Work out the finished part from the listing and answer in its coordinate system (mm). A direction names the side the tool comes from. Give positions to 0.01 mm unless a question says otherwise; leave off trailing zeros. Write each loop counter-clockwise with the first axis right and the second up, starting at its lowest first coordinate (ties: lowest second). Pieces come first, ordered by that corner, then holes.
1) Find section C-C (y = 5). Determine the outline of the cut face in (x, z).
2) Find section B-B (x = 13.75). Determine the outline of the cut face in (y, z), plus the area to 3 significant figures.
3) Find section D-D (x = 18.25). Determine the outline of the cut face in (y, z).
4) Straight lines are drawn through the part: probe 1 along Y at (x, z) = (15, 15.5); probe 2 along Y at (x, z) = (22.25, 23); probe 3 along Z at (x, y) = (18.8, 7.5). For each, find the intervals that lie inside material, in ascending order.
5) Find section A-A (y = 14.5). Determine the outline of the cut face in (x, z).
6) Determine the mould class of faces 1 (the face through (13.943, 20.324, 6.556)), 2 (the face through (16, 9.85, 22)), 3 (the face through (16.278, 6.458, 0.796)) for opening direction X: pulls with the +X half, pulls with the -X half, needs draft (parallel to the pull), parting line crosses it, or undercut.
7) A tool of negligible diameter and unlimited length cuts with its end or side. For faces 4 (the face through (17, 13.1, 0)), 5 (the face through (23.05, 11, 3)), 6 (the face through (14.55, 11, -13)), 7 (the face through (19, 3.3, 24)), 8 (the face through (16, 18.85, 22)), from which of +Z, -Z, +X, -X, +Y, -Y can it reach the whole face along a straight path? Write none if from no direction.
8) Given pin 1 Ø8 at (y, z) = (8, -8) entering from -X; pin 2 Ø9.5 at (y, z) = (6, -15) entering from -X; pin 3 Ø4 at (x, z) = (13.75, 0) entering from -Y; pin 4 Ø4 at (x, y) = (16.5, 6) entering from -Z, each flat-ended and moving along its own axis, determine where each tip first touches the part or whether it passes through.
```python
from build123d import *

# Parameters (mm, degrees)
SKETCH054_R     = 1.7
SKETCH054_R_2   = 2.65
PAD016_DEPTH    = 22
SKETCH055_R     = 9.5
POCKET028_DEPTH = 2.75
POCKET029_DEPTH = 10
POCKET030_DEPTH = 4.5
PAD017_DEPTH    = 22
FILLET046_R     = 3
CHAMFER015_SIZE = 1


with BuildPart() as part:
    # Sketch054 → Pad016 (new body)
    with BuildSketch(Plane.XZ):
        with BuildLine():
            Line((14.55, -17.2), (14.55, -5.5930760767))
            ThreePointArc((14.55, 5.5930760767), (8.1, 0), (14.55, -5.5930760767))
            Line((14.55, 5.5930760767), (14.55, 26))
            Line((14.55, 26), (23.05, 26))
            Line((23.05, 26), (23.05, -17.2))
            ThreePointArc((14.55, -17.2), (18.8, -21.45), (23.05, -17.2))
        make_face()
        with Locations((18.8, -17.2)):
            Circle(SKETCH054_R, mode=Mode.SUBTRACT)
        with Locations((13.75, 0)):
            Circle(SKETCH054_R_2, mode=Mode.SUBTRACT)
    extrude(amount=-PAD016_DEPTH)

    # Sketch055 (on DatumPlane) → Pocket028 (cut, symmetric)
    with BuildSketch(Plane(origin=(6.25, 15.85, 0), x_dir=(0, 0, -1), z_dir=(0, 1, 0))):
        with Locations((0, -7.5)):
            Circle(SKETCH055_R)
    extrude(amount=POCKET028_DEPTH, both=True, mode=Mode.SUBTRACT)

    # Sketch056 (on Face12 of Pocket028) → Pocket029 (cut)
    with BuildSketch(Plane(origin=(23.05, 0, 0), x_dir=(0, 0, 1), z_dir=(1, 0, 0))):
        with BuildLine():
            Line((26, -3.3), (22, -3.3))
            ThreePointArc((22, -3.3), (20.3, -5), (22, -6.7))
            Line((22, -6.7), (26, -6.7))
            Line((26, -6.7), (26, -3.3))
        make_face()
    extrude(amount=-POCKET029_DEPTH, mode=Mode.SUBTRACT)

    # Sketch057 (on DatumPlane) → Pocket030 (cut, symmetric)
    with BuildSketch(Plane(origin=(0, 14.35, 0), x_dir=(1, 0, 0), z_dir=(0, 1, 0))):
        Polygon((14.55, -26), (19.05, -26), (14.55, -10.5), align=None)
    extrude(amount=POCKET030_DEPTH, both=True, mode=Mode.SUBTRACT)

    # Sketch058 (on Face8 of Pocket030) → Pad017 (join)
    with BuildSketch(Plane(origin=(0, 22, 0), x_dir=(1, 0, 0), z_dir=(0, 1, 0))):
        Polygon((23.05, 17.2), (23.05, 18.9604076401), (21.80520382, 20.20520382), align=None)
    extrude(amount=-PAD017_DEPTH)

    # Fillet046
    fillet046_edges = [part.edges().sort_by_distance(p)[0] for p in [
        (14.55, 1.65, 26),
        (14.55, 8.275, 26),
        (14.55, 20.425, 26),
        (14.55, 6.55, 5.593076),
        (14.55, 20.3, 5.593076),
        (14.55, 20.3, -5.593076),
        (14.55, 6.55, -5.593076),
    ]]
    fillet(fillet046_edges, radius=FILLET046_R)

    # Chamfer015
    chamfer015_edges = [part.edges().sort_by_distance(p)[0] for p in [
        (23.05, 1.65, 26),
        (23.05, 14.35, 26),
        (23.05, 15.85, 1.939072),
        (23.05, 15.85, -1.939072),
    ]]
    chamfer(chamfer015_edges, length=CHAMFER015_SIZE)


solid = part.part
```
Results:
1. outline: (12.31, -5.46) arc R3 cw to (14.55, -8.37) - (14.55, -17.2) arc R4.25 ccw to (21.81, -20.21) - (23.05, -18.96) - (23.05, 20.3) - (14.55, 20.3) - (14.55, 8.37) arc R3 cw to (12.31, 5.46) arc R5.65 ccw to start; hole circle Ø5.3 at (13.75, 0); hole circle Ø3.4 at (18.8, -17.2)
2. outline: (0, -6.33) - (13.1, -6.33) - (13.1, -2.65) - (0, -2.65) - close; (0, 2.65) - (13.1, 2.65) - (13.1, 6.33) - (0, 6.33) - close; (18.6, -6.33) - (22, -6.33) - (22, -2.65) - (18.6, -2.65) - close; (18.6, 2.65) - (22, 2.65) - (22, 6.33) - (18.6, 6.33) - close
2. area: 121 mm2
3. outline: (0, -21.41) - (22, -21.41) - (22, -18.81) - (0, -18.81) - close; (0, -15.59) - (22, -15.59) - (22, 26) - (18.85, 26) - (18.85, 23.24) - (9.85, 23.24) - (9.85, 26) - (6.7, 26) - (6.7, 22) arc R1.7 cw to (3.3, 22) - (3.3, 26) - (0, 26) - close; hole (13.1, -8.37) - (18.6, -8.37) - (18.6, 8.37) - (13.1, 8.37) - close
4. probe 1: y = 0 to 9.85, 18.85 to 22
4. probe 2: y = 0 to 3.3, 6.7 to 22
4. probe 3: z = -21.45 to -18.9, -15.5 to 26
5. outline: (14.55, -17.2) arc R4.25 ccw to (21.81, -20.21) - (23.05, -18.96) - (23.05, -2.94) - (22.79, -2.91) arc R9.5 cw to (14.55, -9.47) - close; (14.55, 9.47) arc R9.5 cw to (22.79, 2.91) - (23.05, 2.94) - (23.05, 25) - (22.05, 26) - (19.05, 26) - (14.55, 10.5) - close; hole circle Ø3.4 at (18.8, -17.2)
6. face 1: pulls with the -X half
6. face 2: needs draft
6. face 3: undercut
7. face 4: -X
7. face 5: +Z, -Z, +X, +Y, -Y
7. face 6: -Z, -X, +Y, -Y
7. face 7: +Z, +X, -X
7. face 8: +Z, -X
8. pin 1: stops at x = 9.76
8. pin 2: stops at x = 14.55
8. pin 3: passes through
8. pin 4: stops at z = -21.44
